Autodesk Inventor part; units mm, degrees
ref_plane "YZ Plane" through (0, 0, 0) normal (1, 0, 0) x (0, 1, 0)
ref_plane "XZ Plane" through (0, 0, 0) normal (0, 1, 0) x (-1, 0, 0)
ref_plane "XY Plane" through (0, 0, 0) normal (0, 0, 1) x (1, 0, 0)
ref_plane "Plano de trabalho1" through (0, 0, 0) normal (0, 0, 1) x (1, 0, 0)
sketch "Esboço1" plane through (0, 0, 0) normal (0, 0, 1) x (1, 0, 0)
  circle A0 centre (-15, 0) radius 15
  circle A1 centre (-15, 0) radius 13
  point P0 (0, 0)
  dimension "d0" = 2
extrude "Extrusão1" add sketch "Esboço1" against normal blind 15
sketch "Esboço2" plane through (-15, 0, 0) normal (0, 0, 1) x (1, 0, 0)
  circle A0 centre (0, 0) radius 13
  circle A1 centre (0, 0) radius 20
  circle A2 centre (0, 0) radius 21.5
  point P0 (15, 0)
  dimension "d3" = 43
extrude "Extrusão2" add sketch "Esboço2" along normal blind 5 contours A1 | A2
sketch "Esboço3" plane through (-15, 0, 5) normal (0, 0, 1) x (1, 0, 0)
  circle A0 centre (0, 0) radius 13
  circle A1 centre (0, 0) radius 15
  point P0 (15, 0)
extrude "Extrusão3" add sketch "Esboço3" along normal blind 4
properties part number "Adaptador de Saida"
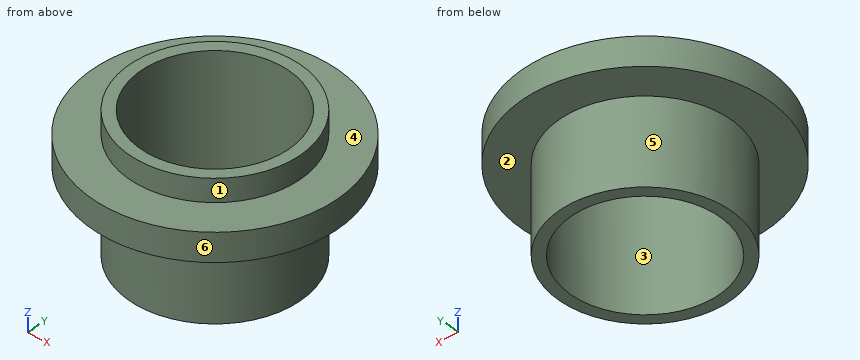
Build history of the part. All positions in model axes, mm. Face numbers are marked on the shaded views. A direction names the side the tool comes from. Give positions to 0.01 mm unless a question says otherwise; leave off trailing zeros. Loops run counter-clockwise (first coordinate to the right, second up) from the corner with the lowest first, then second, coordinate; pieces in that order, holes last. Notation, with made-up numbers: (43, 42) -> (83, 42) arc R24 cw to (83, 76) -> close; hole circle Ø4 at (-15, -0.5). An arc over 180 degrees is marked (long way). One line per question, with ' | ' between items.
Q1. Cut at C-C, the plane z = -5.75. Write the cut outline in (x, y), plus the area to 3 significant figures.
Filled sheet:
outline: circle Ø30 at (-15, 0); hole circle Ø26 at (-15, 0) | area: 176 mm²
Q2. Cut at B-B, the plane y = 0. Write the cut outline in (x, z).
Filled sheet:
outline: (-36.5, 0) -> (-30, 0) -> (-30, -15) -> (-28, -15) -> (-28, 9) -> (-30, 9) -> (-30, 5) -> (-36.5, 5) -> close; (-2, -15) -> (0, -15) -> (0, 0) -> (6.5, 0) -> (6.5, 5) -> (0, 5) -> (0, 9) -> (-2, 9) -> close
Q3. Tool access for the marked faces 4, 5 and 6: list every direction of +Z, -Z, +X, -X, +Y, -Y with a clear straight run to the whole face (end or side of a thin tool).
Filled sheet:
face 4: +Z | face 5: -Z | face 6: +Z, -Z
Q4. Cut at A-A, the plane x = -15. Write the cut outline in (y, z), plus the area to 3 significant figures.
Filled sheet:
outline: (-21.5, 0) -> (-15, 0) -> (-15, -15) -> (-13, -15) -> (-13, 9) -> (-15, 9) -> (-15, 5) -> (-21.5, 5) -> close; (13, -15) -> (15, -15) -> (15, 0) -> (21.5, 0) -> (21.5, 5) -> (15, 5) -> (15, 9) -> (13, 9) -> close | area: 161 mm²
Q5. Drill centre lines: line 1 along Y through (x, z) = (-15, 2.75); line 2 along X through (y, z) = (0.5, -12); line 3 along Y through (x, z) = (-15, -5.25). Where is each one in solid material? Low to high. Write a range as [from, to].
Filled sheet:
line 1: y = [-21.5, -13], [13, 21.5] | line 2: x = [-29.99, -27.99], [-2.01, -0.01] | line 3: y = [-15, -13], [13, 15]
Q6. Drop flat-ended pins along their axis: pin 1 (6 mm diameter, centred on y = 5, z = -11, fed in from -X); pin 2 (1 mm diameter, centred on y = 12.5, z = 0.5, fed in from -X); pin 3 (8 mm diameter, centred on x = -29.5, y = 10.5, fed in from -Z); pin 4 (6 mm diameter, centred on y = 12.5, z = 0.5, fed in from +X). Give the stop position or say it passes through.
Filled sheet:
pin 1: stops at x = -29.87 | pin 2: stops at x = -32.84 | pin 3: stops at z = -15 | pin 4: stops at x = 4.29
Q7. Pull direction X, two halves, no side cores. Call the marked faces 1, 2 and 3: pulls with the +X half, pulls with the -X half, needs draft (parallel to the pull), parting line crosses it, or undercut.
Filled sheet:
face 1: parting line crosses it | face 2: needs draft | face 3: undercut
Q8. Cut at D-D, the plane x = 4. Write the cut outline in (y, z), plus the area to 3 significant figures.
Filled sheet:
outline: (-10.06, 0) -> (10.06, 0) -> (10.06, 5) -> (-10.06, 5) -> close | area: 101 mm²
